The drawing under review shows one solid part. Ordinate dimensions are in mm from its lowest x, y, z. Round coordinates to 2 decimals unless told otherwise and drop trailing zeros. Order: outer loops, then holes, each group sorted by start corner. A loop starts at its lowest first (then second) coordinate and runs counter-clockwise, first axis right, second up. Notation, with made-up numbers: M -0.75,30 L 15.25,30 A21 ccw 15.25,47 Z; hole C 25.5,-31 d8. An arc over 180 degrees is marked long. Answer as a JSON object with one key per item and string values.
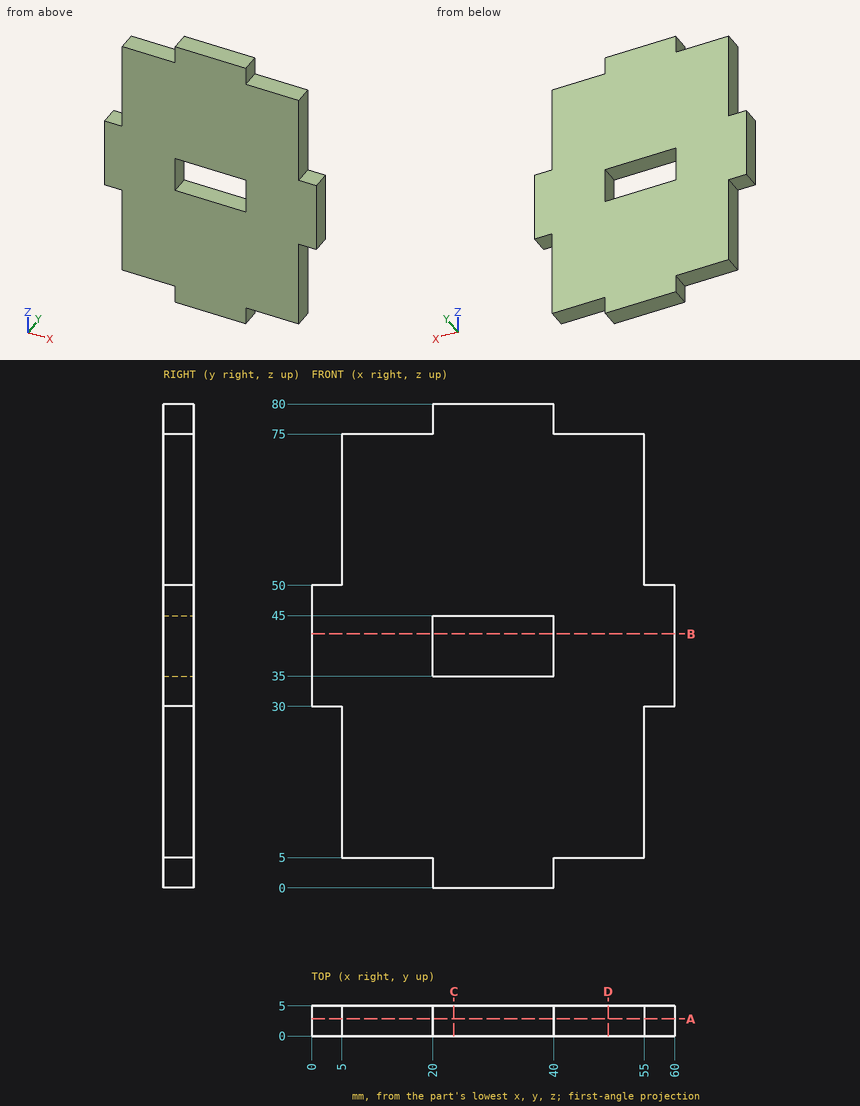
1) Add section D-D on x = 49. State the section outline as (y, z) points, and give its area (3 significant figures).
Geometry check:
{"outline": "M 0,5 L 5,5 L 5,75 L 0,75 Z", "area": "350 mm²"}
2) Add section A-A on y = 2.85. State the section outline as (x, z) points, and give its area (3 significant figures).
Geometry check:
{"outline": "M 0,30 L 5,30 L 5,5 L 20,5 L 20,0 L 40,0 L 40,5 L 55,5 L 55,30 L 60,30 L 60,50 L 55,50 L 55,75 L 40,75 L 40,80 L 20,80 L 20,75 L 5,75 L 5,50 L 0,50 Z; hole M 20,35 L 40,35 L 40,45 L 20,45 Z", "area": "3,700 mm²"}
3) For L1, parallel to Z at x = 31.5, y = 2.9; L2, parallel to Z at x = 46, y = 1.5; L3, parallel to X at y = 3.95, z = 75.5, list the stretches that pass through material, from the lowest coordinate up.
Geometry check:
{"L1": "z = 0 to 35, 45 to 80", "L2": "z = 5 to 75", "L3": "x = 20 to 40"}
4) Add section B-B on z = 42. State the section outline as (x, y) points.
Geometry check:
{"outline": "M 0,0 L 20,0 L 20,5 L 0,5 Z; M 40,0 L 60,0 L 60,5 L 40,5 Z"}
5) Add section C-C on x = 23.5. State the section outline as (y, z) points, and give its area (3 significant figures).
Geometry check:
{"outline": "M 0,0 L 5,0 L 5,35 L 0,35 Z; M 0,45 L 5,45 L 5,80 L 0,80 Z", "area": "350 mm²"}
6) Insertion check: P1, Ø1.5, axis at y = 2, z = 3, coming from the +X side; P2, Ø2.5, axis at y = 3.5, z = 68, coming from the -X side; P3, Ø2.5, axis at y = 3, z = 11.5, coming from the +X side. Each pin has a flat end and moves straight along its axis. Give the tip position at first contact, or say it passes through.
Geometry check:
{"P1": "stops at x = 40", "P2": "stops at x = 5", "P3": "stops at x = 55"}
